```python
from build123d import *

# Parameters (mm, degrees)
F1_DEPTH = 2
F2_R     = 1.375
F3_DEPTH = 2
F4_R     = 1


with BuildPart() as f1:
    # F0 (on Top) → F1 (new body)
    with BuildSketch(Plane.XY):
        with BuildLine():
            ThreePointArc((-34, -2.75), (-32.055456, -1.944544), (-31.25, 0))
            ThreePointArc((-31.25, 0), (-32.055456, 1.944544), (-34, 2.75))
            ThreePointArc((-34, 2.75), (-36.75, 0), (-34, -2.75))
        make_face()
        with BuildLine():
            ThreePointArc((-34, 2.75), (-32.055456, 1.944544), (-31.25, 0))
            ThreePointArc((-31.25, 0), (-32.055456, -1.944544), (-34, -2.75))
            Line((-34, -2.75), (-1.587713, -2.75))
            Line((-1.587713, -2.75), (14.61843, -30.819864))
            ThreePointArc((14.61843, -30.819864), (15.625, -27.063294), (19.38157, -28.069864))
            Line((19.38157, -28.069864), (3.175426, 0))
            Line((3.175426, 0), (19.38157, 28.069864))
            ThreePointArc((19.38157, 28.069864), (15.625, 27.063294), (14.61843, 30.819864))
            Line((14.61843, 30.819864), (-1.587713, 2.75))
            Line((-1.587713, 2.75), (-34, 2.75))
        make_face()
        with BuildLine():
            ThreePointArc((19.75, 29.444864), (17.711752, 32.10116), (14.61843, 30.819864))
            ThreePointArc((14.61843, 30.819864), (15.625, 27.063294), (19.38157, 28.069864))
            ThreePointArc((19.38157, 28.069864), (19.656296, 28.733111), (19.75, 29.444864))
        make_face()
        with BuildLine():
            ThreePointArc((19.38157, -28.069864), (15.625, -27.063294), (14.61843, -30.819864))
            ThreePointArc((14.61843, -30.819864), (17.711752, -32.10116), (19.75, -29.444864))
            ThreePointArc((19.75, -29.444864), (19.656296, -28.733111), (19.38157, -28.069864))
        make_face()
    extrude(amount=F1_DEPTH)

    # F2 (on face) → F3 (cut, through all)
    with BuildSketch(Plane.XY.offset(2)):
        with Locations((-34, 0)):
            Circle(F2_R)
        with Locations((17, 29.444864)):
            Circle(F2_R)
        Circle(F2_R)
        with Locations((17, -29.444864)):
            Circle(F2_R)
    extrude(amount=-F3_DEPTH, mode=Mode.SUBTRACT)

    # F4
    f4_edges = [f1.edges().sort_by_distance(p)[0] for p in [
        (18.375, 31.826434, 2),
        (11.278498, 14.034932, 2),
        (-17.793857, 2.75, 2),
        (6.515358, -16.784932, 2),
    ]]
    fillet(f4_edges, radius=F4_R)


solid = f1.part
```
Check sheet for the modelled part. Datum: model origin and axes. Units: mm. A direction names the side the tool comes from. Round coordinates to 2 decimals unless told otherwise and drop trailing zeros. Loops run counter-clockwise (first coordinate to the right, second up) from the corner with the lowest first, then second, coordinate; pieces in that order, holes last. Notation, with made-up numbers: (20.5, -32) - (61.5, -32) arc R18 cw to (61.5, -27) - close; hole circle Ø7 at (-30.75, 79.25). An arc over 180 degrees is marked (long way). Answer as a JSON object with one key per item and string values. Group by question number.
Q1. Mould release check, pull along Y, two halves, no side actions. Record for faces 4 (the face through (6.516, 16.185, 1.715)), 5 (the face through (6.747, -16.585, 1.715)), 6 (the face through (10.989, 14.135, 1.715)): released by +Y, released by -Y, zero draft, split by the parting line, or undercut.
Q2. Sectioned sample at B-B, the plane x = -11. Enter the section's corners in (y, z), plus the area to 3 significant figures.
Q3. Set-up check for faces 1 (the face through (11.165, 13.838, 0.493)), 2 (the face through (10.758, -13.735, 1.715)), 3 (the face through (6.63, 16.98, 0.49)): record each of +Z, -Z, +X, -X, +Y, -Y from which the full face is reachable in a straight line by a thin tool's end or side.
Q4. Sectioned sample at A-A, the plane z = 0.5. Enter the section's corners in (x, y) (3 decimals).
Q5. Gauge pin test, flat ends, axial feed: P1, Ø0.5, axis at x = -22.5, z = 0.5, coming from the -Y side; P2, Ø2.5, axis at x = -34, y = 0, coming from the +Z side. Record the tip position at first contact, or that the pin passes through.
Q6. Scan lines: line 1 along Y through (x, z) = (17, 1.2); line 2 along Y through (x, z) = (17, 0.55); line 3 along Y through (x, z) = (-1, 1.15). Record each from-to range of solid material in increasing order. Write a range as [from, to].
Solution:
{
 "1": {"face 4": "released by +Y", "face 5": "released by -Y", "face 6": "undercut"},
 "2": {"outline": "(-2.75, 0) - (2.75, 0) - (2.75, 1) arc R1 ccw to (1.75, 2) - (-1.75, 2) arc R1 ccw to (-2.75, 1) - close", "area": "10.6 mm²"},
 "3": {"face 1": "+Z, -Z, +X", "face 2": "+Z, +X", "face 3": "+Z, -Z, -X, +Y"},
 "4": {"outline": "(-34, -2.75) - (-1.588, -2.75) - (14.618, -30.82) arc R2.75 ccw to (19.75, -29.445) arc R2.75 ccw to (19.382, -28.07) - (3.175, 0) - (19.382, 28.07) arc R2.75 ccw to (19.75, 29.445) arc R2.75 ccw to (14.618, 30.82) - (-1.588, 2.75) - (-34, 2.75) arc R2.75 ccw to start; hole circle Ø2.75 at (-34, 0); hole circle Ø2.75 at (0, 0); hole circle Ø2.75 at (17, -29.445); hole circle Ø2.75 at (17, 29.445)"},
 "5": {"P1": "stops at y = -2.75", "P2": "passes through"},
 "6": {"line 1": "y = [-32.17, -30.82], [-28.07, -23.99], [23.99, 28.07], [30.82, 32.17]", "line 2": "y = [-32.19, -30.82], [-28.07, -23.94], [23.94, 28.07], [30.82, 32.19]", "line 3": "y = [-3.75, -0.94], [0.94, 3.75]"}
}
